Geometry: final body of the model. Coordinates: model frame, mm. A direction names the side the tool comes from. Coordinates: 2 decimals unless noted, no trailing zeros. Order: outer loops, then holes, each group sorted by start corner. A loop starts at its lowest first (then second) coordinate and runs counter-clockwise, first axis right, second up. Notation, with made-up numbers: M 11,82 L 21,82 A23 cw 21,99 Z; hole C 71,29.25 d7. An arc over 180 degrees is marked long. Use CSV: the item, a comma, the result in double quotes. Start each with the question number.
1. First-contact query: P1, Ø5, axis at x = 74.5, z = -9.5, coming from the +Y side; P2, Ø2.5, axis at x = 3, z = -22, coming from the +Y side; P3, Ø4, axis at x = 55, z = -18, coming from the +Y side. Flat tips, straight axial feed; report the tip coordinate or a pass-through.
2. Set-up query: faces 1 (the flat face through (38, 8, -27)), 2 (the flat face through (42, 2, -23)), 3 (the flat face through (0, 5, -15)), 4 (the flat face through (73, 10, -15)), 5 (the flat face through (37, 12, -2)). Return all of +Z, -Z, +X, -X, +Y, -Y with unobstructed straight access to the full face (end or side cutting, diameter ignored); none if empty.
3. Material intervals for line 1 (Z direction, x = 73, y = 9); line 2 (X direction, y = 9, z = -22); line 3 (Z direction, x = 47.5, y = 8.5), sorted ascending.
4. Pull-direction query (Z, two-part tool) for faces 6 (the cylindrical face through (3.914, 6.084, -23.433)), 7 (the flat face through (29, 0, -15)), 8 (the flat face through (37, 6, -30)); classes: pulls with the +Z half, pulls with the -Z half, needs draft (parallel to the pull), parting line crosses it, or undercut.
5. Section query D-D on z = -8.25. Return the cut outline in (x, y).
6. Section query A-A on y = 9.5. Return the cut outline in (x, z).
7. Section query C-C on x = 73. Return the cut outline in (y, z).
8. Section query B-B on z = -22. Return the cut outline in (x, y).
from build123d import *

# Parameters (mm, degrees)
SKETCH1_W           = 76
SKETCH1_H           = 30
BOSS_EXTRUDE1_DEPTH = 12
SKETCH2_W           = 64
SKETCH2_H           = 24
CUT_EXTRUDE1_DEPTH  = 9
SKETCH3_R           = 1.7
CUT_EXTRUDE2_DEPTH  = 20
SKETCH4_W           = 6
SKETCH4_H           = 12
CUT_EXTRUDE3_DEPTH  = 5
SKETCH5_W           = 22
SKETCH5_H           = 20
CUT_EXTRUDE4_DEPTH  = 5


with BuildPart() as part:
    # Sketch1 → Boss-Extrude1 (new body)
    with BuildSketch(Plane(origin=(0, 0, 0), x_dir=(1, 0, 0), z_dir=(0, 1, 0))):
        with Locations((38, 15)):
            Rectangle(SKETCH1_W, SKETCH1_H)
    extrude(amount=BOSS_EXTRUDE1_DEPTH)

    # Sketch2 → Cut-Extrude1 (cut)
    with BuildSketch(Plane(origin=(0, 12, 0), x_dir=(1, 0, 0), z_dir=(0, 1, 0))):
        with Locations((38, 15)):
            Rectangle(SKETCH2_W, SKETCH2_H)
    extrude(amount=-CUT_EXTRUDE1_DEPTH, mode=Mode.SUBTRACT)

    # Sketch3 → Cut-Extrude2 (cut)
    with BuildSketch(Plane(origin=(0, 12, 0), x_dir=(1, 0, 0), z_dir=(0, 1, 0))):
        with Locations((73, 22)):
            Circle(SKETCH3_R)
        with Locations((3, 22)):
            Circle(SKETCH3_R)
    extrude(amount=-CUT_EXTRUDE2_DEPTH, mode=Mode.SUBTRACT)

    # Sketch4 → Cut-Extrude3 (cut)
    with BuildSketch(Plane(origin=(0, 12, 0), x_dir=(1, 0, 0), z_dir=(0, 1, 0))):
        with Locations((73, 9)):
            Rectangle(SKETCH4_W, SKETCH4_H)
        with Locations((3, 9)):
            Rectangle(SKETCH4_W, SKETCH4_H)
    extrude(amount=-CUT_EXTRUDE3_DEPTH, mode=Mode.SUBTRACT)

    # Sketch5 → Cut-Extrude4 (cut)
    with BuildSketch(Plane(origin=(0, 3, 0), x_dir=(1, 0, 0), z_dir=(0, 1, 0))):
        with Locations((42, 13)):
            Rectangle(SKETCH5_W, SKETCH5_H)
    extrude(amount=-CUT_EXTRUDE4_DEPTH, mode=Mode.SUBTRACT)


solid = part.part
Results list:
1,P1,"stops at y = 7"
1,P2,"passes through"
1,P3,"stops at y = 3"
2,face 1,"+Y"
2,face 2,"+Y, -Y"
2,face 3,"+Z, -Z, -X, +Y, -Y"
2,face 4,"+X, -X, +Y"
2,face 5,"+Z, -Z, +X, -X, +Y"
3,line 1,"z = -30 to -23.7, -20.3 to -15, -3 to 0"
3,line 2,"x = 0 to 1.3, 4.7 to 6, 70 to 71.3, 74.7 to 76"
3,line 3,"z = -30 to -27, -3 to 0"
4,face 6,"undercut"
4,face 7,"needs draft"
4,face 8,"pulls with the -Z half"
5,outline,"M 0,0 L 31,0 L 31,3 L 6,3 L 6,7 L 0,7 Z; M 53,0 L 76,0 L 76,7 L 70,7 L 70,3 L 53,3 Z"
6,outline,"M 0,-30 L 76,-30 L 76,-15 L 70,-15 L 70,-27 L 6,-27 L 6,-15 L 0,-15 Z; M 0,-3 L 76,-3 L 76,0 L 0,0 Z; hole C 3,-22 d3.4; hole C 73,-22 d3.4"
7,outline,"M 0,-30 L 12,-30 L 12,-23.7 L 0,-23.7 Z; M 0,-20.3 L 12,-20.3 L 12,-15 L 7,-15 L 7,-3 L 12,-3 L 12,0 L 0,0 Z"
8,outline,"M 0,0 L 1.3,0 L 1.3,12 L 0,12 Z; M 4.7,0 L 31,0 L 31,3 L 6,3 L 6,12 L 4.7,12 Z; M 53,0 L 71.3,0 L 71.3,12 L 70,12 L 70,3 L 53,3 Z; M 74.7,0 L 76,0 L 76,12 L 74.7,12 Z"
